Here's how the part is built. I have some questions about the finished solid (model axes, mm). A direction names the side the tool comes from. Give positions to 0.01 mm unless a question says otherwise; leave off trailing zeros. Loops run counter-clockwise (first coordinate to the right, second up) from the corner with the lowest first, then second, coordinate; pieces in that order, holes last. Notation, with made-up numbers: (1, 85.25) - (59, 85.25) arc R19 cw to (59, 120.25) - close; hole circle Ø2 at (-15, -37). An arc over 180 degrees is marked (long way). Return JSON: item names as keys, results as strings. Group by question number.
(1) If we section it at C-C (x = 60): Please give me the cut outline in (y, z), then the cut area to 4 significant figures.
(2) If we section it at D-D (z = -60): Please give me the cut outline in (x, y), then the cut area to 4 significant figures.
(3) On a 3-axis mill with a long thin cutter (end or side, diameter ignored), from which of +Z, -Z, +X, -X, +Y, -Y can I reach the whole of each face in a straight line? I mean faces 4 (the flat face through (-1, 0, -1)), 5 (the flat face through (-1, 5, -70)), 6 (the flat face through (1, 6.8, -22)). Say none if no direction works.
(4) If we mould it in two halves opening along Z, with no side actions, what happens to faces 1 (the flat face through (-1, 0, 62)), 2 (the cylindrical face through (17.09, 8.38, -22.14)), 3 (the cylindrical face through (-11.923, -2.465, 53.692))? For each: released by +Z, released by -Z, zero draft, split by the parting line, or undercut.
(5) I need wall thicknesses on probe 1 along Z at (x, y) = (60, 3); probe 2 along Z at (x, y) = (-62.5, 3.25) (3 decimals); probe 3 along Z at (x, y) = (0, 8.55). Which ranges of each line are inside material? Lowest first, please. Write a range as [from, to].
(6) If we section it at B-B (z = 0): State how many separate pieces and enclosed holes the cut face has, then the cut area to 3 significant figures.
(7) If we section it at A-A (x = 0): Please give me the cut outline in (y, z), then the cut area to 3 significant figures.
(8) For P1, Ø8, axis at x = 17.68, z = 17.68, coming from the -Y side; P2, Ø8, axis at x = 0, z = 25, coming from the +Y side; P3, Ø1, axis at y = -1, z = 27, coming from the +X side, each with a flat end and sliding along its axis, tell me the tip position at first contact or that it passes through.
```python
from build123d import *

# Parameters (mm, degrees)
SKETCH1_W           = 130
SKETCH1_H           = 160
SKETCH1_R           = 4.5
BOSS_EXTRUDE1_DEPTH = 10
SKETCH1_8_R         = 55
SKETCH1_8_R_2       = 45
BOSS_EXTRUDE2_DEPTH = 5
SKETCH1_9_R         = 4.5
SKETCH1_9_R_2       = 3
BOSS_EXTRUDE3_DEPTH = 6.8
SKETCH4_R           = 1.6
CUT_EXTRUDE1_DEPTH  = 10
SKETCH5_R           = 2.25
CUT_EXTRUDE2_DEPTH  = 10


with BuildPart() as part:
    # Sketch1 → Boss-Extrude1 (new body)
    with BuildSketch(Plane(origin=(0, 0, 0), x_dir=(1, 0, 0), z_dir=(0, 1, 0))):
        with Locations((0, -10)):
            Rectangle(SKETCH1_W, SKETCH1_H)
        with Locations((17.67766953, 17.67766953)):
            Circle(SKETCH1_R, mode=Mode.SUBTRACT)
        with Locations((25, 0)):
            Circle(SKETCH1_R, mode=Mode.SUBTRACT)
        with Locations((-17.67766953, -17.67766953)):
            Circle(SKETCH1_R, mode=Mode.SUBTRACT)
        with Locations((0, -25)):
            Circle(SKETCH1_R, mode=Mode.SUBTRACT)
        with Locations((17.67766953, -17.67766953)):
            Circle(SKETCH1_R, mode=Mode.SUBTRACT)
        with Locations((-25, 0)):
            Circle(SKETCH1_R, mode=Mode.SUBTRACT)
        with Locations((-17.67766953, 17.67766953)):
            Circle(SKETCH1_R, mode=Mode.SUBTRACT)
        with Locations((0, 25)):
            Circle(SKETCH1_R, mode=Mode.SUBTRACT)
    extrude(amount=BOSS_EXTRUDE1_DEPTH)

    # Sketch1<8> → Boss-Extrude2 (add)
    with BuildSketch(Plane(origin=(0, 0, 0), x_dir=(1, 0, 0), z_dir=(0, 1, 0))):
        Circle(SKETCH1_8_R)
        Circle(SKETCH1_8_R_2, mode=Mode.SUBTRACT)
    extrude(amount=-BOSS_EXTRUDE2_DEPTH)

    # Sketch1<9> → Boss-Extrude3 (add)
    with BuildSketch(Plane(origin=(0, 0, 0), x_dir=(1, 0, 0), z_dir=(0, 1, 0))):
        with Locations((17.67766953, -17.67766953)):
            Circle(SKETCH1_9_R)
        with Locations((17.67766953, -17.67766953)):
            Circle(SKETCH1_9_R_2, mode=Mode.SUBTRACT)
        with Locations((25, 0)):
            Circle(SKETCH1_9_R)
        with Locations((25, 0)):
            Circle(SKETCH1_9_R_2, mode=Mode.SUBTRACT)
        with Locations((17.67766953, 17.67766953)):
            Circle(SKETCH1_9_R)
        with Locations((17.67766953, 17.67766953)):
            Circle(SKETCH1_9_R_2, mode=Mode.SUBTRACT)
        with Locations((0, 25)):
            Circle(SKETCH1_9_R)
        with Locations((0, 25)):
            Circle(SKETCH1_9_R_2, mode=Mode.SUBTRACT)
        with Locations((-17.67766953, 17.67766953)):
            Circle(SKETCH1_9_R)
        with Locations((-17.67766953, 17.67766953)):
            Circle(SKETCH1_9_R_2, mode=Mode.SUBTRACT)
        with Locations((-25, 0)):
            Circle(SKETCH1_9_R)
        with Locations((-25, 0)):
            Circle(SKETCH1_9_R_2, mode=Mode.SUBTRACT)
        with Locations((-17.67766953, -17.67766953)):
            Circle(SKETCH1_9_R)
        with Locations((-17.67766953, -17.67766953)):
            Circle(SKETCH1_9_R_2, mode=Mode.SUBTRACT)
        with Locations((0, -25)):
            Circle(SKETCH1_9_R)
        with Locations((0, -25)):
            Circle(SKETCH1_9_R_2, mode=Mode.SUBTRACT)
    extrude(amount=BOSS_EXTRUDE3_DEPTH)

    # Sketch4 → Cut-Extrude1 (cut)
    with BuildSketch(Plane(origin=(0, 10, 0), x_dir=(1, 0, 0), z_dir=(0, 1, 0))):
        with Locations((-62.5, 65)):
            Circle(SKETCH4_R)
        with Locations((-62.5, 8.655)):
            Circle(SKETCH4_R)
        with Locations((-62.5, -47.69)):
            Circle(SKETCH4_R)
    extrude(amount=-CUT_EXTRUDE1_DEPTH, mode=Mode.SUBTRACT)

    # Sketch5 → Cut-Extrude2 (cut)
    with BuildSketch(Plane(origin=(0, 10, 0), x_dir=(1, 0, 0), z_dir=(0, 1, 0))):
        with Locations((60, 60)):
            Circle(SKETCH5_R)
        with Locations((60, 0)):
            Circle(SKETCH5_R)
        with Locations((60, -60)):
            Circle(SKETCH5_R)
    extrude(amount=-CUT_EXTRUDE2_DEPTH, mode=Mode.SUBTRACT)


solid = part.part
```
Values:
{
 "1": {"outline": "(0, -70) - (10, -70) - (10, -62.25) - (0, -62.25) - close; (0, -57.75) - (10, -57.75) - (10, -2.25) - (0, -2.25) - close; (0, 2.25) - (10, 2.25) - (10, 57.75) - (0, 57.75) - close; (0, 62.25) - (10, 62.25) - (10, 90) - (0, 90) - close", "area": "1,465 mm2"},
 "2": {"outline": "(-65, 0) - (57.75, 0) - (57.75, 10) - (-65, 10) - close; (62.25, 0) - (65, 0) - (65, 10) - (62.25, 10) - close", "area": "1,255 mm2"},
 "3": {"face 4": "-Y", "face 5": "-Z, +X, -X, +Y, -Y", "face 6": "+Y"},
 "4": {"face 1": "zero draft", "face 2": "undercut", "face 3": "split by the parting line"},
 "5": {"probe 1": "[-70, -62.25], [-57.75, -2.25], [2.25, 57.75], [62.25, 90]", "probe 2": "[-70, -66.6], [-63.4, -10.255], [-7.055, 46.09], [49.29, 90]", "probe 3": "[-70, -29.5], [-20.5, 20.5], [29.5, 90]"},
 "6": {"separate pieces": "4", "enclosed holes": "0", "area": "1,220 mm2"},
 "7": {"outline": "(-5, -55) - (0, -55) - (0, -70) - (10, -70) - (10, -29.5) - (6.8, -29.5) - (6.8, -28) - (0, -28) - (0, -45) - (-5, -45) - close; (-5, 45) - (0, 45) - (0, 28) - (6.8, 28) - (6.8, 29.5) - (10, 29.5) - (10, 90) - (0, 90) - (0, 55) - (-5, 55) - close; (0, -22) - (6.8, -22) - (6.8, -20.5) - (10, -20.5) - (10, 20.5) - (6.8, 20.5) - (6.8, 22) - (0, 22) - close", "area": "1,560 mm2"},
 "8": {"P1": "y = 0", "P2": "y = 6.8", "P3": "x = 48.19"}
}
